```python
from build123d import *

# Parameters (mm, degrees)
SKETCH1_W           = 15.24
SKETCH1_H           = 15.24
BOSS_EXTRUDE1_DEPTH = 3.81
BOSS_EXTRUDE2_DEPTH = 1.6002
SKETCH3_W           = 15.24
SKETCH3_H           = 15.24
BOSS_EXTRUDE3_DEPTH = 3.81
SKETCH4_R           = 1.778
CUT_EXTRUDE1_DEPTH  = 15.851000211
FILLET1_R           = 0.762


with BuildPart() as part:
    # Sketch1 → Boss-Extrude1 (new body)
    with BuildSketch(Plane(origin=(0, 0, 0), x_dir=(1, 0, 0), z_dir=(0, 1, 0))):
        with Locations((-1.182029268, 0)):
            Rectangle(SKETCH1_W, SKETCH1_H)
    extrude(amount=BOSS_EXTRUDE1_DEPTH)

    # Sketch2 → Boss-Extrude2 (add)
    with BuildSketch(Plane(origin=(0, 3.81, 0), x_dir=(1, 0, 0), z_dir=(0, 1, 0))):
        Polygon((-8.802029268, -2.54), (-3.722029268, -2.54), (-3.722029268, -7.62), (6.437970732, -7.62), (6.437970732, 7.62), (-8.802029268, 7.62), align=None)
    extrude(amount=BOSS_EXTRUDE2_DEPTH)

    # Sketch3 → Boss-Extrude3 (add)
    with BuildSketch(Plane(origin=(0, 5.4102, 0), x_dir=(1, 0, 0), z_dir=(0, 1, 0))):
        with Locations((-1.182029268, 0)):
            Rectangle(SKETCH3_W, SKETCH3_H)
    extrude(amount=BOSS_EXTRUDE3_DEPTH)

    # Sketch4 → Cut-Extrude1 (cut, through all)
    with BuildSketch(Plane(origin=(0, 9.2202, 0), x_dir=(1, 0, 0), z_dir=(0, 1, 0))):
        with Locations(Location((3.262970732, 4.445, 0), (0, 0, 270))):
            Circle(SKETCH4_R)
    extrude(amount=-CUT_EXTRUDE1_DEPTH, mode=Mode.SUBTRACT)

    # Fillet1
    fillet1_edges = [part.edges().sort_by_distance(p)[0] for p in [
        (-8.802029268, 9.2202, 0),
        (-1.182029268, 9.2202, 7.62),
        (6.437970732, 9.2202, 0),
        (-1.182029268, 9.2202, -7.62),
    ]]
    fillet(fillet1_edges, radius=FILLET1_R)


solid = part.part
```
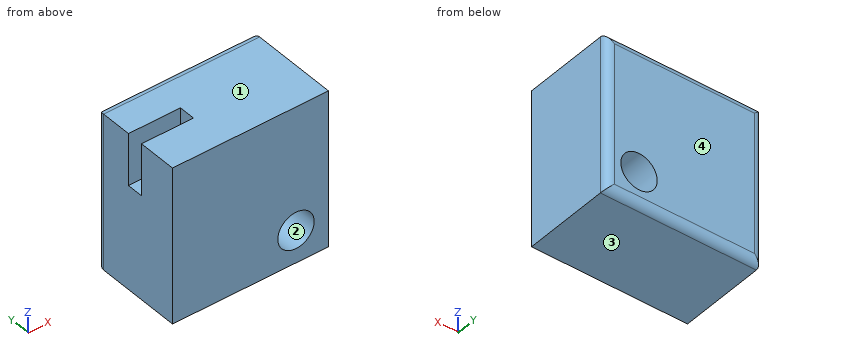
Here's how the part is built. I have some questions about the finished solid (model axes, mm). Face numbers are marked on the shaded views. Give positions to 0.01 mm unless a question says otherwise; leave off trailing zeros. Loops run counter-clockwise (first coordinate to the right, second up) from the corner with the lowest first, then second, coordinate; pieces in that order, holes last. Notation, with made-up numbers: M 79.5,83 L 126.5,83 A7 cw 126.5,93 Z; hole C -6.5,-27 d4. An arc over 180 degrees is marked long. Return JSON: item names as keys, results as strings.
Item 1: Imagine slicing it at C-C on y = 1.5. List the corners of the cut face in (x, z) for me (3 decimals), then the cut area to 3 significant figures.
A:
{"outline": "M -8.802,-7.62 L 6.438,-7.62 L 6.438,7.62 L -8.802,7.62 Z; hole C 3.263,-4.445 d3.556", "area": "222 mm^2"}
Item 2: Imagine slicing it at A-A on z = 3.5. List the corners of the cut face in (x, y) for me, then the cut area to 3 significant figures.
A:
{"outline": "M -8.8,0 L 6.44,0 L 6.44,8.46 A0.76 ccw 5.68,9.22 L -8.04,9.22 A0.76 ccw -8.8,8.46 L -8.8,5.41 L -3.72,5.41 L -3.72,3.81 L -8.8,3.81 Z", "area": "132 mm^2"}
Item 3: Please list where these lines run through material, in increasing order: line 1 (Y direction, x = 5.75, z = 3.25); line 2 (Y direction, x = -5.5, z = 4.75); line 3 (Z direction, x = 2.5, y = 4.5).
A:
{"line 1": "y = 0 to 9.22", "line 2": "y = 0 to 3.81, 5.41 to 9.22", "line 3": "z = -7.62 to -6.05, -2.84 to 7.62"}
Item 4: I'm going to push flat-ended pins straight in: pin 1 Ø0.5 at (y, z) = (4.5, 5) entering from -X; pin 2 Ø3 at (x, z) = (3.26, -4.44) entering from -Y. Where does each tip first touch, or does it pass through?
A:
{"pin 1": "stops at x = -3.72", "pin 2": "passes through"}
Item 5: Thinking about a two-plate mould opening in Z: for the marked faces 1, 2, 3 and 4, which applies, released by +Z, released by -Z, zero draft, split by the parting line, or undercut?
A:
{"face 1": "released by +Z", "face 2": "undercut", "face 3": "released by -Z", "face 4": "zero draft"}
Item 6: Imagine slicing it at D-D on z = -5.25. List the corners of the cut face in (x, y) for me.
A:
{"outline": "M -8.8,0 L 1.68,0 L 1.68,9.22 L -8.04,9.22 A0.76 ccw -8.8,8.46 Z; M 4.85,0 L 6.44,0 L 6.44,8.46 A0.76 ccw 5.68,9.22 L 4.85,9.22 Z"}
Item 7: Imagine slicing it at B-B on x = 2.75. List the corners of the cut face in (y, z) for me, then the cut area to 3 significant figures.
A:
{"outline": "M 0,-7.62 L 8.46,-7.62 A0.76 ccw 9.22,-6.86 L 9.22,-6.15 L 0,-6.15 Z; M 0,-2.74 L 9.22,-2.74 L 9.22,6.86 A0.76 ccw 8.46,7.62 L 0,7.62 Z", "area": "109 mm^2"}
